from build123d import *

# Parameters (mm, degrees)
BOSS_EXTRUDE1_DEPTH       = 13.2
F_1_5MM_DOWEL_HOLE1_D     = 1.5
F_1_5MM_DOWEL_HOLE1_DEPTH = 6
F_1_5MM_DOWEL_HOLE1_TIP   = 0.450645464
F_1_5MM_DOWEL_HOLE7_D     = 1.5
F_1_5MM_DOWEL_HOLE7_DEPTH = 6
F_1_5MM_DOWEL_HOLE7_TIP   = 0.450645464


with BuildPart() as part:
    # Sketch3 → Boss-Extrude1 (new body)
    with BuildSketch(Plane(origin=(0, 0, 0), x_dir=(0, 0, -1), z_dir=(1, 0, 0))):
        Polygon((0, 0), (13.2, 0), (13.2, 5), (13.2, 5.9), (7.9, 5.9), (7.9, 5), (0, 5), align=None)
    extrude(amount=BOSS_EXTRUDE1_DEPTH)

    # Ø1.5mm Dowel Hole1
    with Locations(Plane(origin=(0, 0, -13.2), x_dir=(-1, 0, 0), z_dir=(0, 0, -1))):
        with Locations((-3.6, 2.95)):
            Hole(F_1_5MM_DOWEL_HOLE1_D / 2, depth=F_1_5MM_DOWEL_HOLE1_DEPTH)
            with Locations((0, 0, -(F_1_5MM_DOWEL_HOLE1_DEPTH + F_1_5MM_DOWEL_HOLE1_TIP / 2))):  # 118° drill point
                Cone(0, F_1_5MM_DOWEL_HOLE1_D / 2, F_1_5MM_DOWEL_HOLE1_TIP, mode=Mode.SUBTRACT)

    # Ø1.5mm Dowel Hole7
    with Locations(Plane(origin=(0, 0, -13.2), x_dir=(-1, 0, 0), z_dir=(0, 0, -1))):
        with Locations((-9.6, 2.95)):
            Hole(F_1_5MM_DOWEL_HOLE7_D / 2, depth=F_1_5MM_DOWEL_HOLE7_DEPTH)
            with Locations((0, 0, -(F_1_5MM_DOWEL_HOLE7_DEPTH + F_1_5MM_DOWEL_HOLE7_TIP / 2))):  # 118° drill point
                Cone(0, F_1_5MM_DOWEL_HOLE7_D / 2, F_1_5MM_DOWEL_HOLE7_TIP, mode=Mode.SUBTRACT)


solid = part.part
Geometry: final body of the model. Coordinates: model frame, mm. A direction names the side the tool comes from. Coordinates: 2 decimals unless noted, no trailing zeros. Loops run counter-clockwise (first coordinate to the right, second up) from the corner with the lowest first, then second, coordinate; pieces in that order, holes last. Notation, with made-up numbers: (-38.75, 67) - (-29.75, 67) arc R21 ccw to (-29.75, 85) - close; hole circle Ø2 at (-40, 25). An arc over 180 degrees is marked (long way). Put each result on its own line as item: value. Start each with the question number.
Q1. Cut plane D-D, the plane z = -9. Return loops of the section in (x, y), and give its area (3 significant figures).
Q2. Set-up query: faces 1 (the cylindrical face through (9.502, 3.694, -10.158)), 2 (the flat face through (7, 3, 0)), 3 (the flat face through (6.5, 5.5, -7.9)). Return all of +Z, -Z, +X, -X, +Y, -Y with unobstructed straight access to the full face (end or side cutting, diameter ignored); none if empty.
Q3. Cut plane C-C, the plane z = -2.75. Return loops of the section in (x, y), and give its area (3 significant figures).
Q4. Line query: line 1 (X direction, y = 2.95, z = -8.7); line 2 (Y direction, x = 3.6, z = -10.2); line 3 (X direction, y = 2.85, z = -7). Output: solid intervals per line, ascending.
Q5. Cut plane B-B, the plane x = 11.25. Return loops of the section in (y, z).
Q6. Pin query (flat end, axial travel): pin 1 Ø0.5 at (x, y) = (5, 5.5) entering from +Z; pin 2 Ø1.4 at (x, y) = (3.6, 2.95) entering from -Z; pin 3 Ø1.2 at (x, y) = (9.6, 2.95) entering from -Z. Return the tip coordinate at first contact, or that it passes through.
Q7. Cut plane A-A, the plane z = -7.5. Return loops of the section in (x, y).
Q8. Pull-direction query (X, two-part tool) for faces 4 (the flat face through (0, 3, -7)), 5 (the flat face through (7, 3, -13.2)), 6 (the conical face through (3.703, 2.871, -6.828)); classes: released by +X, released by -X, zero draft, split by the parting line, or undercut.
Filled sheet:
1. outline: (0, 0) - (13.2, 0) - (13.2, 5.9) - (0, 5.9) - close; hole circle Ø1.5 at (3.6, 2.95); hole circle Ø1.5 at (9.6, 2.95)
1. area: 74.3 mm²
2. face 1: -Z
2. face 2: +Z, +X, -X, +Y, -Y
2. face 3: +Z, +X, -X, +Y
3. outline: (0, 0) - (13.2, 0) - (13.2, 5) - (0, 5) - close
3. area: 66.0 mm²
4. line 1: 0 to 2.85, 4.35 to 8.85, 10.35 to 13.2
4. line 2: 0 to 2.2, 3.7 to 5.9
4. line 3: 0 to 3.2, 4 to 9.2, 10 to 13.2
5. outline: (0, -13.2) - (5.9, -13.2) - (5.9, -7.9) - (5, -7.9) - (5, 0) - (0, 0) - close
6. pin 1: z = -7.9
6. pin 2: z = -7.17
6. pin 3: z = -7.11
7. outline: (0, 0) - (13.2, 0) - (13.2, 5) - (0, 5) - close; hole circle Ø1.5 at (3.6, 2.95); hole circle Ø1.5 at (9.6, 2.95)
8. face 4: released by -X
8. face 5: zero draft
8. face 6: undercut
